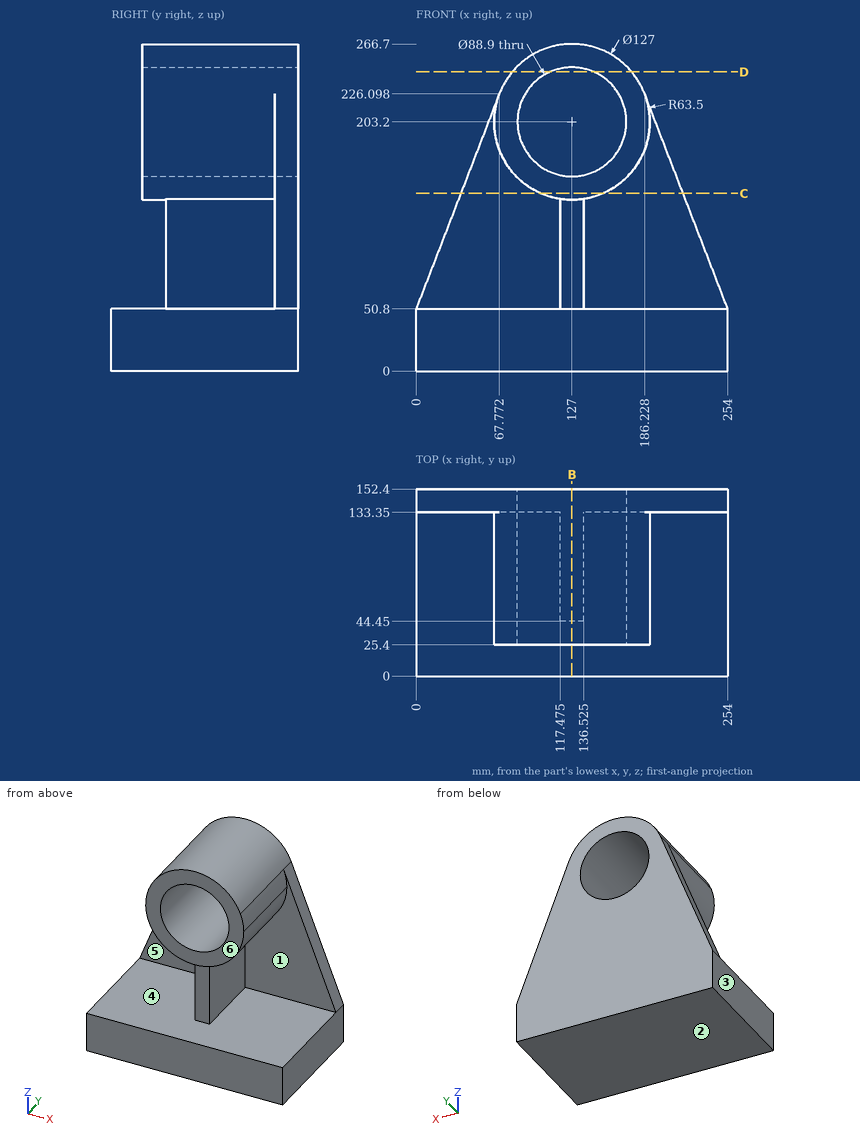
Geometry check sheet. Reference: drawing and pictorial views, mm from the part's lowest x, y, z. A direction names the side the tool comes from. Give positions to 0.01 mm unless a question says otherwise; leave off trailing zeros. Order: outer loops, then holes, each group sorted by start corner. A loop starts at its lowest first (then second) coordinate and runs counter-clockwise, first axis right, second up.
1. Section check C-C, the plane z = 145. Enter the section's corners in (x, y), and give its area (3 significant figures).
2. Section check D-D, the plane z = 244. Enter the section's corners in (x, y), and give its area (3 significant figures).
3. Thickness scan on L1, parallel to Z at x = 127, y = 125; L2, parallel to Y at x = 86.5, z = 102; L3, parallel to Z at x = 164.5, y = 54 (1 decimal). Record the ranges inside material, lowest first.
4. Release check for a two-part mould opening along Z. For the marked faces 1, 2 and 3 record: pulls with the +Z half, pulls with the -Z half, needs draft (parallel to the pull), parting line crosses it, or undercut.
5. Section check B-B, the plane x = 127. Enter the section's corners in (y, z), and give its area (3 significant figures).
6. Gauge pin test, flat ends, axial feed: pin 1 Ø1 at (x, y) = (179, 49.5) entering from +Z; pin 2 Ø2 at (x, y) = (196.5, 72) entering from +Z; pin 3 Ø3 at (y, z) = (53.5, 148) entering from -X; pin 4 Ø1.5 at (y, z) = (32, 138.5) entering from +X. Record the tip position at first contact, or that the pin passes through.
7. Access from +Z, -Z, +X, -X, +Y, -Y to the whole of each face (thin tool, end or side, straight path). Record for the marked faces 4, 5 and 6.
Values follow:
1. outline: (36.42, 133.35) - (101.6, 133.35) - (101.6, 25.4) - (152.4, 25.4) - (152.4, 133.35) - (217.58, 133.35) - (217.58, 152.4) - (36.42, 152.4) - close
1. area: 8,930 mm2
2. outline: (78.34, 25.4) - (109.36, 25.4) - (109.36, 152.4) - (78.34, 152.4) - close; (144.64, 25.4) - (175.66, 25.4) - (175.66, 152.4) - (144.64, 152.4) - close
2. area: 7,880 mm2
3. L1: z = 0 to 158.75, 247.65 to 266.7
3. L2: y = 133.35 to 152.4
3. L3: z = 0 to 50.8, 152 to 179.3, 227.1 to 254.4
4. face 1: undercut
4. face 2: pulls with the -Z half
4. face 3: needs draft
5. outline: (0, 0) - (152.4, 0) - (152.4, 158.75) - (25.4, 158.75) - (25.4, 139.7) - (44.45, 139.7) - (44.45, 50.8) - (0, 50.8) - close; (25.4, 247.65) - (152.4, 247.65) - (152.4, 266.7) - (25.4, 266.7) - close
5. area: 22,200 mm2
6. pin 1: stops at z = 240.35
6. pin 2: stops at z = 50.8
6. pin 3: stops at x = 93.11
6. pin 4: passes through
7. face 4: -Y
7. face 5: -X, -Y
7. face 6: +Z, +X, -X, -Y
